The model under review builds one solid part; all positions refer to its coordinate system, in mm. Round coordinates to 2 decimals unless told otherwise and drop trailing zeros. Loops run counter-clockwise (first coordinate to the right, second up) from the corner with the lowest first, then second, coordinate; pieces in that order, holes last. Notation, with made-up numbers: M 66,72.25 L 99,72.25 A29 cw 99,105.25 Z; hole C 79,-15.75 d2. An arc over 180 degrees is marked long. Return JSON: item names as keys, results as strings. Group by question number.
Q1. To check wall thickness, follow line 1 along Z through (x, y) = (0, 16); line 2 along Z through (x, y) = (0, 6.5); line 3 along X through (y, z) = (18.5, -54). State the ranges of each line that lie inside material, in increasing order.
Q2. Clearance check with flat-ended pins moving along their axes: pin 1 Ø4 at (y, z) = (17.5, -86.5) entering from +X; pin 2 Ø4 at (y, z) = (7.5, 16.5) entering from -X; pin 3 Ø4 at (x, y) = (-106, 4.5) entering from -Z. State where each tip first meets the part, or that it passes through.
Q3. Consider section B-B (z = 0). State the section outline as (x, y) points (3 decimals).
Q4. Draft analysis for pull direction Z (two halves, no side actions). For faces 1 (the face through (119.8, 0, -94.5)), 2 (the face through (-120.94, 10.39, -92.73)), 3 (the face through (-127.49, 0.386, -97.756)), state which applies: pulls with the +Z half, pulls with the -Z half, needs draft (parallel to the pull), parting line crosses it, or undercut.
Q5. Consider section A-A (x = 0). State the section outline as (y, z) points (3 decimals), and give its area (3 significant figures).
from build123d import *

# Parameters (mm, degrees)
FILLET1_R     = 0.508
CHAMFER1_SIZE = 0.508


with BuildPart() as part:
    # Sketch1 → Revolve1 (revolve)
    with BuildSketch(Plane.XY):
        Polygon((152.4, 21.082), (152.4, 0), (160.655, 0), (160.655, 0.762), (159.639, 0.762), (159.639, 10.922), (152.908, 10.922), (152.908, 19.686281471), align=None)
    revolve(axis=Axis((0, 28.738956579, 0), (0, -1, 0)))

    # Fillet1
    fillet1_edges = [part.edges().sort_by_distance(p)[0] for p in [
        (-159.639, 0.762, 0),
        (-152.908, 10.922, 0),
    ]]
    fillet(fillet1_edges, radius=FILLET1_R)

    # Chamfer1
    chamfer1_edges = [part.edges().sort_by_distance(p)[0] for p in [
        (-159.639, 10.922, 0),
    ]]
    chamfer(chamfer1_edges, length=CHAMFER1_SIZE)


solid = part.part
Values:
{
 "1": {"line 1": "z = -152.91 to -152.4, 152.4 to 152.91", "line 2": "z = -159.64 to -152.4, 152.4 to 159.64", "line 3": "x = -143.06 to -142.51, 142.51 to 143.06"},
 "2": {"pin 1": "stops at x = 127.44", "pin 2": "stops at x = -158.98", "pin 3": "stops at z = -121.11"},
 "3": {"outline": "M -160.655,0 L -152.4,0 L -152.4,21.082 L -152.908,19.686 L -152.908,11.43 A0.508 cw -153.416,10.922 L -159.131,10.922 L -159.639,10.414 L -159.639,1.27 A0.508 cw -160.147,0.762 L -160.655,0.762 Z; M 152.4,0 L 160.655,0 L 160.655,0.762 L 160.147,0.762 A0.508 cw 159.639,1.27 L 159.639,10.414 L 159.131,10.922 L 153.416,10.922 A0.508 cw 152.908,11.43 L 152.908,19.686 L 152.4,21.082 Z"},
 "4": {"face 1": "needs draft", "face 2": "undercut", "face 3": "parting line crosses it"},
 "5": {"outline": "M 0,-160.655 L 0.762,-160.655 L 0.762,-160.147 A0.508 cw 1.27,-159.639 L 10.414,-159.639 L 10.922,-159.131 L 10.922,-153.416 A0.508 cw 11.43,-152.908 L 19.686,-152.908 L 21.082,-152.4 L 0,-152.4 Z; M 0,152.4 L 21.082,152.4 L 19.686,152.908 L 11.43,152.908 A0.508 cw 10.922,153.416 L 10.922,159.131 L 10.414,159.639 L 1.27,159.639 A0.508 cw 0.762,160.147 L 0.762,160.655 L 0,160.655 Z", "area": "169 mm2"}
}
